Could you check a few things on this model? Use its own coordinates, in mm. A direction names the side the tool comes from. Round coordinates to 2 decimals unless told otherwise and drop trailing zeros. Loops run counter-clockwise (first coordinate to the right, second up) from the corner with the lowest first, then second, coordinate; pieces in that order, holes last. Notation, with made-up numbers: (32.25, -7.75) -> (65.25, -7.75) arc R11 ccw to (65.25, 3.25) -> close; hole circle Ø11 at (-16, 25). An arc over 180 degrees is marked (long way). Write each question's results on one line, items separated by ' | '. Start each with the question number.
1) For P1, Ø1.1, axis at x = 0.5, z = 1.5, coming from the +Y side; P2, Ø1.9, axis at x = -3.96, y = 11.5, coming from the +Z side; P3, Ø0.7, axis at x = 15.5, z = 1.5, coming from the -Y side; P4, Ø1.1, axis at y = 17, z = 1.5, coming from the -X side, each with a flat end and sliding along its axis, tell me the tip position at first contact or that it passes through.
2) Imagine slicing it at B-B, the plane z = 1.15. Give the number of separate pieces and of enclosed holes in the cut face, plus the area to 3 significant figures.
3) Imagine slicing it at C-C, the plane x = 15. List the corners of the cut face in (y, z) for me.
4) Which directions (+Z, -Z, +X, -X, +Y, -Y) give clear straight access to the entire face, cutting with the end or side of a thin tool? Please do faces 5 (the flat face through (0, 6.5, 1)), 6 (the flat face through (0, 15.3, 1)), 7 (the flat face through (15, -7.5, 1)), 8 (the flat face through (14, 13, 1)).
5) If I drill on probe 1 along Y at (x, z) = (5, 1.95); probe 2 along Y at (x, z) = (-3.5, 0.3); probe 3 along Y at (x, z) = (-5, 0.2), over which ranges is the centre line in solid material (lowest first)?
6) We'd pull the mould along X, two halves only. Please class faces 1 (the flat face through (-9, 0, 1)), 2 (the cylindrical face through (3.117, 14.295, 1.085)), 3 (the flat face through (9, 17.5, 1)), 4 (the flat face through (14, -11, 1)): pulls with the +X half, pulls with the -X half, needs draft (parallel to the pull), parting line crosses it, or undercut.
7) Imagine slicing it at A-A, the plane y = 11.5. List the corners of the cut face in (x, z) for me, plus the area to 3 significant figures.
8) Imagine slicing it at D-D, the plane y = 2.5. List the corners of the cut face in (x, z) for me.
from build123d import *

# Parameters (mm, degrees)
SKETCH_1_R      = 1.55
SKETCH_1_W      = 18
SKETCH_1_H      = 13
EXTRUDE_1_DEPTH = 2.2
CHAMFER_1_SIZE  = 6


with BuildPart() as part:
    # 草图1 → 凸台-拉伸1 (new body)
    with BuildSketch(Plane.XY):
        with BuildLine():
            Line((-14, -17.5), (14, -17.5))
            Line((14, -17.5), (14, -9.51))
            ThreePointArc((14, -9.51), (12.995, -8.505), (14, -7.5))
            Line((14, -7.5), (17, -7.5))
            Line((17, -7.5), (17, 7.5))
            Line((17, 7.5), (14, 7.5))
            ThreePointArc((14, 7.5), (12.995, 8.505), (14, 9.51))
            Line((14, 9.51), (14, 17.5))
            Line((14, 17.5), (4.1, 17.5))
            Line((4.1, 17.5), (4.1, 15.3))
            ThreePointArc((4.1, 15.3), (3.095, 14.295), (2.09, 15.3))
            Line((2.09, 15.3), (-2.09, 15.3))
            ThreePointArc((-2.09, 15.3), (-3.095, 14.295), (-4.1, 15.3))
            Line((-4.1, 15.3), (-4.1, 17.5))
            Line((-4.1, 17.5), (-14, 17.5))
            Line((-14, 17.5), (-14, 9.51))
            ThreePointArc((-14, 9.51), (-13.289357685, 9.215642315), (-12.995, 8.505))
            ThreePointArc((-12.995, 8.505), (-13.289357685, 7.794357685), (-14, 7.5))
            Line((-14, 7.5), (-17, 7.5))
            Line((-17, 7.5), (-17, -7.5))
            Line((-17, -7.5), (-14, -7.5))
            ThreePointArc((-14, -7.5), (-13.289357685, -7.794357685), (-12.995, -8.505))
            ThreePointArc((-12.995, -8.505), (-13.289357685, -9.215642315), (-14, -9.51))
            Line((-14, -9.51), (-14, -17.5))
        make_face()
        with Locations((2.882843865, -11.677628522)):
            Circle(SKETCH_1_R, mode=Mode.SUBTRACT)
        Rectangle(SKETCH_1_W, SKETCH_1_H, mode=Mode.SUBTRACT)
        with Locations((-3.958028601, 11.5)):
            Circle(SKETCH_1_R, mode=Mode.SUBTRACT)
    extrude(amount=EXTRUDE_1_DEPTH)

    # 倒角1
    chamfer_1_edges = [part.edges().sort_by_distance(p)[0] for p in [
        (14, -17.5, 1.1),
        (-14, -17.5, 1.1),
    ]]
    chamfer(chamfer_1_edges, length=CHAMFER_1_SIZE)


solid = part.part
Checked values:
1) P1: y = 15.3 | P2: through | P3: y = -7.5 | P4: x = -14
2) separate pieces: 1 | enclosed holes: 3 | area: 757 mm^2
3) outline: (-7.5, 0) -> (7.5, 0) -> (7.5, 2.2) -> (-7.5, 2.2) -> close
4) face 5: +Z, -Z | face 6: +Z, -Z, +Y | face 7: +Z, -Z, +X, -Y | face 8: +Z, -Z, +X, +Y
5) probe 1: -17.5 to -6.5, 6.5 to 17.5 | probe 2: -17.5 to -6.5, 6.5 to 10.02, 12.98 to 14.38 | probe 3: -17.5 to -6.5, 6.5 to 10.35, 12.65 to 17.5
6) face 1: undercut | face 2: undercut | face 3: needs draft | face 4: pulls with the +X half
7) outline: (-14, 0) -> (-5.51, 0) -> (-5.51, 2.2) -> (-14, 2.2) -> close; (-2.41, 0) -> (14, 0) -> (14, 2.2) -> (-2.41, 2.2) -> close | area: 54.8 mm^2
8) outline: (-17, 0) -> (-9, 0) -> (-9, 2.2) -> (-17, 2.2) -> close; (9, 0) -> (17, 0) -> (17, 2.2) -> (9, 2.2) -> close
